Geometry check sheet. Reference: the model listing, model coordinates, mm. Face numbers are marked on the shaded views. Give positions to 0.01 mm unless a question says otherwise; leave off trailing zeros. Loops run counter-clockwise (first coordinate to the right, second up) from the corner with the lowest first, then second, coordinate; pieces in that order, holes last. Notation, with made-up numbers: (71.25, 27) -> (85.25, 27) arc R27 cw to (85.25, 61) -> close; hole circle Ø11 at (-2.5, 79). An arc over 180 degrees is marked (long way). Answer in a Markdown table with one row per item. Add a question column.
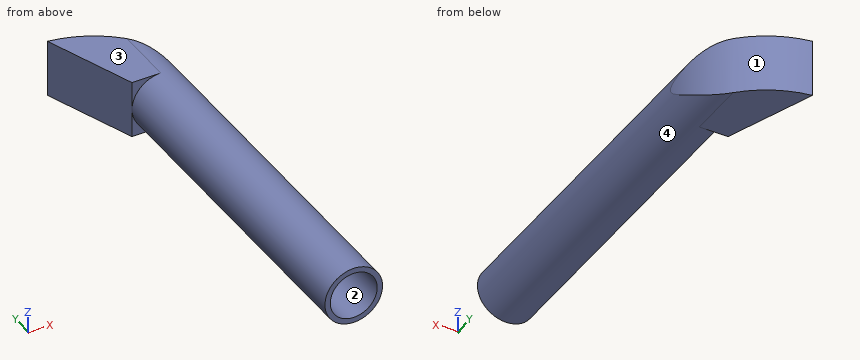
```python
from build123d import *

# Parameters (mm, degrees)
SKETCH1_R                = 13.5
SKETCH1_R_2              = 11
BOSS_EXTRUDE1_DEPTH      = 152.4
SKETCH2_R                = 13.5
BOSS_EXTRUDE2_DEPTH      = 5
BOSS_EXTRUDE3_DEPTH      = 15
BOSS_EXTRUDE3_DEPTH_BACK = 15
CUT_EXTRUDE3_DEPTH       = 60


with BuildPart() as part:
    # Sketch1 → Boss-Extrude1 (new body)
    with BuildSketch(Plane(origin=(0, 0, 0), x_dir=(1, 0, 0), z_dir=(0, 1, 0))):
        with Locations(Location((0, 0, 0), (0, 0, 90))):
            Circle(SKETCH1_R)
        with Locations(Location((0, 0, 0), (0, 0, 90))):
            Circle(SKETCH1_R_2, mode=Mode.SUBTRACT)
    extrude(amount=BOSS_EXTRUDE1_DEPTH)

    # Sketch2 → Boss-Extrude2 (add)
    with BuildSketch(Plane(origin=(0, 152.4, 0), x_dir=(1, 0, 0), z_dir=(0, 1, 0))):
        with Locations(Location((0, 0, 0), (0, 0, 90))):
            Circle(SKETCH2_R)
    extrude(amount=BOSS_EXTRUDE2_DEPTH)

    # Sketch4 → Boss-Extrude3 (add, two sides: drawn at the far end of the back side and taken through both)
    with BuildSketch(Plane.XY.offset(-BOSS_EXTRUDE3_DEPTH_BACK)):
        with BuildLine():
            Line((-11.023106702708283, 157.4), (13.500000000000005, 157.4))
            ThreePointArc((13.500000000000005, 157.4), (-0.5561486693953412, 185.6697206774346), (-28.92642808378068, 199.52178437011307))
            Line((-28.92642808378068, 199.52178437011307), (-13.5, 157.4))
            Line((-13.5, 157.4), (-11.023106702708283, 157.4))
        make_face()
    extrude(amount=BOSS_EXTRUDE3_DEPTH + BOSS_EXTRUDE3_DEPTH_BACK)

    # Sketch6 → Cut-Extrude3 (cut)
    with BuildSketch(Plane.XZ.offset(-157.4)):
        with BuildLine():
            Line((1.65e-15, -13.5), (-22.83152492307377, -13.5))
            Line((-22.83152492307377, -13.5), (-32.31073418001762, -13.5))
            Line((-32.31073418001762, -13.5), (-41.11350108400584, -13.5))
            Line((-41.11350108400584, -13.5), (-41.11350108400584, -20.862107506591272))
            Line((-41.11350108400584, -20.862107506591272), (-22.42358054940404, -20.091260403237417))
            Line((-22.42358054940404, -20.091260403237417), (15.387763585115868, -20.091260403237417))
            Line((15.387763585115868, -20.091260403237417), (15.387763585115868, 20.065763879883022))
            Line((15.387763585115868, 20.065763879883022), (-22.42358054940404, 20.065763879883022))
            Line((-22.42358054940404, 20.065763879883022), (-41.11350108400584, 20.065763879883022))
            Line((-41.11350108400584, 20.065763879883022), (-41.55310392760487, 13.317013583252685))
            Line((-41.55310392760487, 13.317013583252685), (-30.569316507300755, 13.499999999999883))
            Line((-30.569316507300755, 13.499999999999883), (-5.044e-14, 13.499999999999998))
            ThreePointArc((-5.044e-14, 13.499999999999998), (13.5, 2.398e-14), (1.65e-15, -13.5))
        make_face()
    extrude(amount=-CUT_EXTRUDE3_DEPTH, mode=Mode.SUBTRACT)


solid = part.part
```
1. Release check for a two-part mould opening along X. For the marked faces 1, 2, 3 and 4 record: released by +X, released by -X, zero draft, split by the parting line, or undercut.
2. Sectioned sample at B-B (z = -7). Enter the section's corners in (x, y).
3. Material ranges on L1, parallel to X at y = 110.5, z = 0; L2, parallel to Z at x = -2.5, y = 104; L3, parallel to X at y = 128, z = -7.5, recorded low to high. Write a range as from..to.
4. Sectioned sample at A-A (y = 147). Enter the section's corners in (x, z).
5. Sectioned sample at D-D (z = 4). Enter the section's corners in (x, y), plus the area to 3 significant figures.
6. Gauge pin test, flat ends, axial feed: pin 1 Ø1.5 at (x, z) = (3.5, -4) entering from -Y; pin 2 Ø11 at (x, z) = (-6.5, -6) entering from -Y; pin 3 Ø3 at (x, z) = (-7, -3) entering from +Y; pin 4 Ø1.5 at (y, z) = (122.5, 3.5) entering from +X. Record the tip position at first contact, or that the pin passes through.
7. Sectioned sample at C-C (x = 2.5). Enter the section's corners in (y, z).
Response:
| question | item | result |
|---|---|---|
| 1 | face 1 | released by +X |
| 1 | face 2 | undercut |
| 1 | face 3 | zero draft |
| 1 | face 4 | split by the parting line |
| 2 | outline | (-28.93, 199.52) -> (-13.5, 157.4) -> (-11.54, 157.4) -> (-11.54, 0) -> (-8.49, 0) -> (-8.49, 152.4) -> (8.49, 152.4) -> (8.49, 0) -> (11.54, 0) -> (11.54, 166) arc R49.06 ccw to start |
| 3 | L1 | x = -13.5..-11, 11..13.5 |
| 3 | L2 | z = -13.27..-10.71, 10.71..13.27 |
| 3 | L3 | x = -11.22..-8.05, 8.05..11.22 |
| 4 | outline | circle Ø27 at (0, 0); hole circle Ø22 at (0, 0) |
| 5 | outline | (-28.93, 199.52) -> (-13.5, 157.4) -> (-12.89, 157.4) -> (-12.89, 0) -> (-10.25, 0) -> (-10.25, 152.4) -> (10.25, 152.4) -> (10.25, 0) -> (12.89, 0) -> (12.89, 160.93) arc R49.06 ccw to start |
| 5 | area | 1,920 mm2 |
| 6 | pin 1 | stops at y = 152.4 |
| 6 | pin 2 | stops at y = 0 |
| 6 | pin 3 | stops at y = 192.06 |
| 6 | pin 4 | stops at x = 13.22 |
| 7 | outline | (0, -13.27) -> (182.34, -13.27) -> (182.34, 13.27) -> (0, 13.27) -> (0, 10.71) -> (152.4, 10.71) -> (152.4, -10.71) -> (0, -10.71) -> close |
